Build history of the part. All positions in model axes, mm. Face numbers are marked on the shaded views. A direction names the side the tool comes from. Give positions to 0.01 mm unless a question says otherwise; leave off trailing zeros. Order: outer loops, then holes, each group sorted by start corner. A loop starts at its lowest first (then second) coordinate and runs counter-clockwise, first axis right, second up. Notation, with made-up numbers: (79.25, -13) - (93.25, -13) arc R28 ccw to (93.25, 9) - close; hole circle Ø1 at (45.5, 55.5). An arc over 180 degrees is marked (long way). Write each question's results on one line, items separated by ' | '. Start each with the question number.
1) Tool access for the marked faces 4 and 5: list every direction of +Z, -Z, +X, -X, +Y, -Y with a clear straight run to the whole face (end or side of a thin tool).
2) Cut at A-A on y = 47. List the corners of the cut face in (x, z), plus the area to 3 significant figures.
3) Cut at B-B on z = -64. State how many separate pieces and enclosed holes the cut face has, plus the area to 3 significant figures.
4) Drill centre lines: line 1 along Y through (x, z) = (16, -65); line 2 along X through (y, z) = (97, -44); line 3 along Y through (x, z) = (84, -80). Where is each one in solid material? Low to high. Write a range as from..to.
5) Two-plate mould, pull along Y, no slides. Class the marked faces 1, 2 and 3: +Y half, -Y half, draft (parallel to the pull), parting line (faces both ways), or undercut.
6) Cut at C-C on y = 171. List the corners of the cut face in (x, z), plus the area to 3 significant figures.
7) Drop flat-ended pins along their axis: pin 1 Ø2.5 at (y, z) = (116, -105.5) entering from -X; pin 2 Ø13.5 at (x, z) = (108.33, -108.33) entering from +Y; pin 3 Ø3 at (y, z) = (346, -69) entering from -X; pin 4 Ø6.5 at (x, z) = (8.33, -108.33) entering from +Y. Give the stop position or say it passes through.
from build123d import *

# Parameters (mm, degrees)
SKETCH1_W                = 350
SKETCH1_H                = 350
BOSS_EXTRUDE1_DEPTH      = 50
FILLET1_R                = 25
SKETCH2_R                = 12.5
CUT_EXTRUDE1_DEPTH       = 50
SKETCH3_R                = 150
BOSS_EXTRUDE2_DEPTH      = 300
FILLET2_R                = 15
CHAMFER1_SIZE            = 15
SKETCH5_W                = 135
SKETCH5_H                = 135
CUT_EXTRUDE3_DEPTH       = 90
SCALE1_SCALE             = 0.333333333
EXTRUDE_THIN1_DEPTH      = 250
EXTRUDE_THIN1_DEPTH_BACK = 5
BOSS_EXTRUDE3_START      = -15
SKETCH7_R                = 50
BOSS_EXTRUDE3_DEPTH      = 15
SKETCH8_W                = 25.5
SKETCH8_H                = 25.5
CUT_EXTRUDE4_DEPTH       = 9.5
SKETCH9_W                = 65
SKETCH9_H                = 100
CUT_EXTRUDE5_DEPTH       = 6
SKETCH10_W               = 10
SKETCH10_H               = 23.333333333
CUT_EXTRUDE6_DEPTH       = 378.683913993
SKETCH12_R               = 37.5
CUT_EXTRUDE7_DEPTH       = 75


with BuildPart() as part:
    # Sketch1 → Boss-Extrude1 (new body)
    with BuildSketch(Plane(origin=(0, 0, 0), x_dir=(1, 0, 0), z_dir=(0, 1, 0))):
        with Locations((175, 175)):
            Rectangle(SKETCH1_W, SKETCH1_H)
    extrude(amount=-BOSS_EXTRUDE1_DEPTH)

    # Fillet1
    fillet1_edges = [part.edges().sort_by_distance(p)[0] for p in [
        (0, -25, -350),
        (350, -25, -350),
        (350, -25, 0),
        (0, -25, 0),
    ]]
    fillet(fillet1_edges, radius=FILLET1_R)

    # Sketch2 → Cut-Extrude1 (cut)
    with BuildSketch(Plane(origin=(0, 0, 0), x_dir=(1, 0, 0), z_dir=(0, 1, 0))):
        with Locations(Location((25, 25, 0), (0, 0, 270))):
            Circle(SKETCH2_R)
        with Locations(Location((325, 25, 0), (0, 0, 270))):
            Circle(SKETCH2_R)
        with Locations(Location((325, 325, 0), (0, 0, 270))):
            Circle(SKETCH2_R)
        with Locations(Location((25, 325, 0), (0, 0, 270))):
            Circle(SKETCH2_R)
    extrude(amount=-CUT_EXTRUDE1_DEPTH, mode=Mode.SUBTRACT)

    # Sketch3 → Boss-Extrude2 (add)
    with BuildSketch(Plane(origin=(0, 0, 0), x_dir=(1, 0, 0), z_dir=(0, 1, 0))):
        with Locations(Location((175, 175, 0), (0, 0, 90))):
            Circle(SKETCH3_R)
    extrude(amount=BOSS_EXTRUDE2_DEPTH)

    # Fillet2
    fillet2_edges = [part.edges().sort_by_distance(p)[0] for p in [
        (175, 0, -25),
    ]]
    fillet(fillet2_edges, radius=FILLET2_R)

    # Chamfer1
    chamfer1_edges = [part.edges().sort_by_distance(p)[0] for p in [
        (175, 300, -25),
    ]]
    chamfer(chamfer1_edges, length=CHAMFER1_SIZE)

    # Sketch5 → Cut-Extrude3 (cut)
    with BuildSketch(Plane.XZ.offset(-300)):
        with Locations((175, -175)):
            Rectangle(SKETCH5_W, SKETCH5_H)
    extrude(amount=CUT_EXTRUDE3_DEPTH, mode=Mode.SUBTRACT)


with BuildPart() as part_1:
    # Scale1: scaled about (0, 0, 0)
    add(part.part.scale(SCALE1_SCALE))

    # Sketch6 → Extrude-Thin1 (add, two sides: drawn at the far end of the back side and taken through both)
    with BuildSketch(Plane(origin=(0, 100, 0), x_dir=(1, 0, 0), z_dir=(0, 1, 0)).offset(-EXTRUDE_THIN1_DEPTH_BACK)):
        with BuildLine():
            ThreePointArc((48.391261826, 107.334917126), (74.830545561, 105.5333544), (96.635555489, 90.472713818))
            Line((96.635555489, 90.472713818), (92.805333274, 87.258775769))
            ThreePointArc((92.805333274, 87.258775769), (73.180824339, 100.813352293), (49.385468977, 102.434758746))
            Line((49.385468977, 102.434758746), (48.391261826, 107.334917126))
        make_face()
    extrude(amount=EXTRUDE_THIN1_DEPTH + EXTRUDE_THIN1_DEPTH_BACK)

    # Sketch7 → Boss-Extrude3 (add)
    with BuildSketch(Plane(origin=(0, 350, 0), x_dir=(1, 0, 0), z_dir=(0, 1, 0)).offset(BOSS_EXTRUDE3_START)):
        with Locations(Location((58.333333333, 58.333333333, 0), (0, 0, 90))):
            Circle(SKETCH7_R)
    extrude(amount=BOSS_EXTRUDE3_DEPTH)

    # Sketch8 → Cut-Extrude4 (cut)
    with BuildSketch(Plane.XZ.offset(-335)):
        with Locations((58.333333333, -58.333333333)):
            Rectangle(SKETCH8_W, SKETCH8_H)
    extrude(amount=-CUT_EXTRUDE4_DEPTH, mode=Mode.SUBTRACT)

    # Sketch9 → Cut-Extrude5 (cut)
    with BuildSketch(Plane(origin=(0, 350, 0), x_dir=(1, 0, 0), z_dir=(0, 1, 0))):
        with Locations((58.333333333, 58.333333333)):
            Rectangle(SKETCH9_W, SKETCH9_H)
    extrude(amount=-CUT_EXTRUDE5_DEPTH, mode=Mode.SUBTRACT)

    # Sketch10 → Cut-Extrude6 (cut, through all)
    with BuildSketch(Plane.XY.offset(-80.833333333)):
        with Locations((59.575622215, 111.666666667)):
            Rectangle(SKETCH10_W, SKETCH10_H)
    extrude(amount=-CUT_EXTRUDE6_DEPTH, mode=Mode.SUBTRACT)

    # Sketch12 → Cut-Extrude7 (cut)
    with BuildSketch(Plane(origin=(0, -16.666666667, 0), x_dir=(1, 0, 0), z_dir=(0, 1, 0))):
        with Locations(Location((58.333333333, 58.333333333, 0), (0, 0, 270))):
            Circle(SKETCH12_R)
    extrude(amount=CUT_EXTRUDE7_DEPTH, mode=Mode.SUBTRACT)


solid = part_1.part
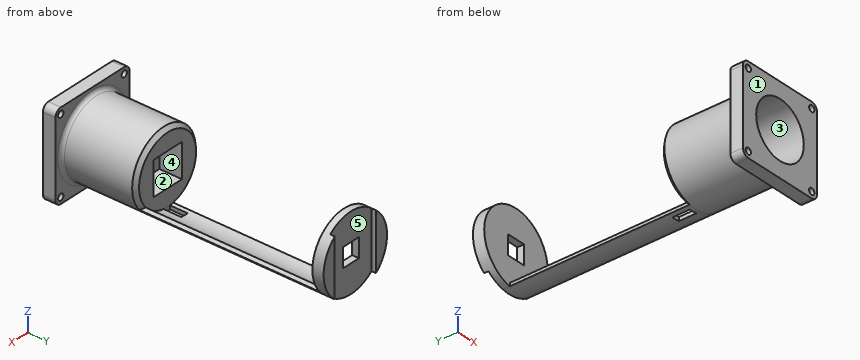
Results:
1) face 4: none | face 5: +Z, -Z, +Y
2) outline: circle Ø100 at (58.33, -58.33); hole circle Ø75 at (58.33, -58.33) | area: 3,440 mm^2
3) separate pieces: 3 | enclosed holes: 0 | area: 5,830 mm^2
4) line 1: -16.67..100, 335..350 | line 2: 12.52..35.83, 80.83..104.14 | line 3: 58.33..100, 335..344
5) face 1: -Y half | face 2: undercut | face 3: draft
6) outline: (48.39, -107.33) arc R50 ccw to (96.64, -90.47) - (92.81, -87.26) arc R45 cw to (49.39, -102.43) - close | area: 255 mm^2
7) pin 1: x = 48.51 | pin 2: y = 0 | pin 3: x = 9.18 | pin 4: through
